Could you check a few things on this model? Use its own coordinates, in mm. A direction names the side the tool comes from. Coordinates: 2 decimals unless noted, no trailing zeros. Loops run counter-clockwise (first coordinate to the right, second up) from the corner with the lowest first, then second, coordinate; pieces in that order, holes last. Notation, with made-up numbers: M 53.25,-30 L 86.25,-30 A19 ccw 86.25,-6 Z; hole C -5.75,58 d1. An arc over 180 degrees is marked long. Use one line per item in the form item = value. Start each with the question number.
```python
from build123d import *

# Parameters (mm, degrees)
SKETCH1_R           = 2.4
SKETCH1_R_2         = 5
BOSS_EXTRUDE1_DEPTH = 5
SKETCH2_R           = 5
SKETCH2_R_2         = 1
BOSS_EXTRUDE2_DEPTH = 3
SKETCH3_R           = 2
CUT_EXTRUDE1_DEPTH  = 1


with BuildPart() as part:
    # Sketch1 → Boss-Extrude1 (new body)
    with BuildSketch(Plane(origin=(0, 0, 0), x_dir=(0.999713496, 0.023935854, 0), z_dir=(0, 0, 1))):
        with BuildLine():
            Line((10.010039278, 5.570210903), (10.010039278, 49.980040959))
            ThreePointArc((10.010039278, 49.980040959), (5.010039278, 54.980040959), (0.010039278, 49.980040959))
            Line((0.010039278, 49.980040959), (0.010039278, 5.570210903))
            ThreePointArc((0.010039278, 5.570210903), (5.010039278, -7.519959041), (10.010039278, 5.570210903))
        make_face()
        with Locations((5.010039278, 49.980040959)):
            Circle(SKETCH1_R, mode=Mode.SUBTRACT)
        with Locations((5.010039278, -0.019959041)):
            Circle(SKETCH1_R_2, mode=Mode.SUBTRACT)
    extrude(amount=BOSS_EXTRUDE1_DEPTH)

    # Sketch2 → Boss-Extrude2 (add)
    with BuildSketch(Plane.XY.offset(5)):
        with Locations((3.812288906, 50.085641068)):
            Circle(SKETCH2_R)
        with Locations((3.812288906, 50.085641068)):
            Circle(SKETCH2_R_2, mode=Mode.SUBTRACT)
    extrude(amount=BOSS_EXTRUDE2_DEPTH)

    # Sketch3 → Cut-Extrude1 (cut)
    with BuildSketch(Plane.XY.offset(8)):
        with Locations((3.812288906, 50.085641068)):
            Circle(SKETCH3_R)
    extrude(amount=-CUT_EXTRUDE1_DEPTH, mode=Mode.SUBTRACT)


solid = part.part
```
Item 1: For faces 1 (the cylindrical face through (5, 48, 2)), 2 (the flat face through (3, 51, 7)), 3 (the flat face through (6, 50, 8)), which set-ups out of +Z, -Z, +X, -X, +Y, -Y let a thin tool reach every point of the face, with its end or its side?
Item 2: Thinking about a two-plate mould opening in Y: for faces 4 (the flat face through (6, 24, 0)), 5 (the cylindrical face through (3.55, 52.07, 7.51)), which applies, pulls with the +Y half, pulls with the -Y half, needs draft (parallel to the pull), parting line crosses it, or undercut?
Item 3: I'm going to push flat-ended pins straight in: P1, Ø4, axis at x = 3.81, y = 50.09, coming from the -Z side; P2, Ø3, axis at x = 9, z = 6.5, coming from the +Y side; P3, Ø4.5, axis at x = 8.5, y = 35.5, coming from the +Z side. Where does each tip first touch, or does it pass through?
Item 4: I want a section at D-D (y = 24). Write out the boundary of the cut face in (x, z), plus the area to 3 significant figures.
Item 5: I want a section at A-A (x = 3.75). Write out the boundary of the cut face in (y, z).
Item 6: I want a section at C-C (z = 1). Write out the boundary of the cut face in (x, y).
Item 7: I want a section at B-B (y = -3). Write out the boundary of the cut face in (x, z), plus the area to 3 significant figures.
Item 8: Please list where these lines run through material, in increasing order: line 1 along Z through (x, y) = (-0.25, 2); line 2 along Y through (x, z) = (5.75, 2); line 3 along Y through (x, z) = (3, 1.5).
Worked answers:
q1.face_1 = -Z
q1.face_2 = +Z
q1.face_3 = +Z, +X, -X, +Y, -Y
q2.face_4 = needs draft
q2.face_5 = undercut
q3.P1 = 5
q3.P2 = 53.46
q3.P3 = 5
q4.outline = M -0.56,0 L 9.44,0 L 9.44,5 L -0.56,5 Z
q4.area = 50.0 mm²
q5.outline = M -7.29,0 L -4.74,0 L -4.74,5 L -7.29,5 Z; M 4.94,0 L 47.69,0 L 47.69,5 L 49.09,5 L 49.09,7 L 48.09,7 L 48.09,8 L 45.09,8 L 45.09,5 L 4.94,5 Z; M 51.08,5 L 52.48,5 L 52.48,0 L 55.09,0 L 55.09,8 L 52.08,8 L 52.08,7 L 51.08,7 Z
q6.outline = M -1.19,49.97 L -0.12,5.57 A7.5 ccw long 9.87,5.81 L 8.81,50.21 A5 ccw Z; hole C 5.01,0.1 d10; hole C 3.81,50.09 d4.8
q7.outline = M -1.82,0 L 1.09,0 L 1.09,5 L -1.82,5 Z; M 8.93,0 L 11.84,0 L 11.84,5 L 8.93,5 Z
q7.area = 29.1 mm²
q8.line_1 = 0 to 5
q8.line_2 = -7.36 to -4.84, 5.04 to 48.67, 51.5 to 54.69
q8.line_3 = -7.13 to -4.48, 4.68 to 47.83, 52.34 to 55.02
